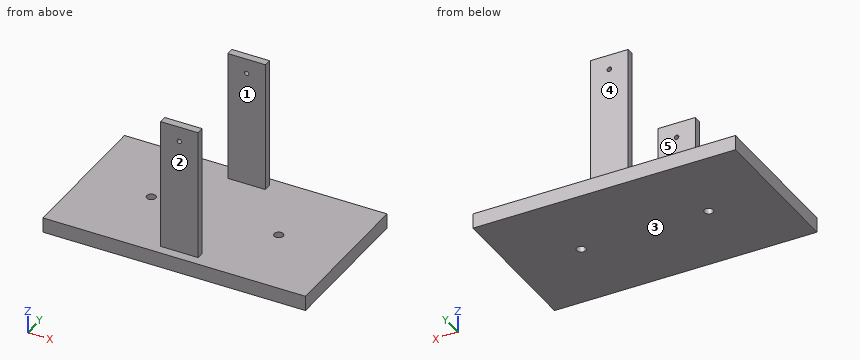
```python
from build123d import *

# Parameters (mm, degrees)
SKETCH_W        = 70
SKETCH_H        = 40
PAD_DEPTH       = 4
SKETCH001_W     = 10
SKETCH001_H     = 2
PAD001_DEPTH    = 35
SKETCH002_R     = 0.6
POCKET_DEPTH    = 37
SKETCH003_R     = 1.2
POCKET001_DEPTH = 5


with BuildPart() as part:
    # Sketch → Pad (new body)
    with BuildSketch(Plane.XY):
        with Locations((35, 20)):
            Rectangle(SKETCH_W, SKETCH_H)
    extrude(amount=PAD_DEPTH)

    # Sketch001 (on Face6 of Pad) → Pad001 (join)
    with BuildSketch(Plane.XY.offset(4)):
        with Locations((35, 36.5)):
            Rectangle(SKETCH001_W, SKETCH001_H)
        with Locations((35, 3.5)):
            Rectangle(SKETCH001_W, SKETCH001_H)
    extrude(amount=PAD001_DEPTH)

    # Sketch002 (on Face8 of Pad001) → Pocket (cut)
    with BuildSketch(Plane.XZ.offset(-2.5)):
        with Locations((35, 35)):
            Circle(SKETCH002_R)
    extrude(amount=-POCKET_DEPTH, mode=Mode.SUBTRACT)

    # Sketch003 (on Face4 of Pocket) → Pocket001 (cut)
    with BuildSketch(Plane(origin=(0, 0, 0), x_dir=(1, 0, 0), z_dir=(0, 0, -1))):
        with Locations((18, -20)):
            Circle(SKETCH003_R)
        with Locations((52, -20)):
            Circle(SKETCH003_R)
    extrude(amount=-POCKET001_DEPTH, mode=Mode.SUBTRACT)


solid = part.part
```
Geometry: final body of the model. Coordinates: model frame, mm. Face numbers are marked on the shaded views. A direction names the side the tool comes from. Coordinates: 2 decimals unless noted, no trailing zeros. Loops run counter-clockwise (first coordinate to the right, second up) from the corner with the lowest first, then second, coordinate; pieces in that order, holes last. Notation, with made-up numbers: M 47.5,-19 L 92.5,-19 A22 cw 92.5,13 Z; hole C -23.75,-14.75 d9. An arc over 180 degrees is marked long. Put each result on its own line as item: value.
(1) Access query for the marked faces 4 and 5. Directions: +Z, -Z, +X, -X, +Y, -Y. A direction counts if a zero-diameter tool reaches every point of the face in a straight line with its end or side. Return the directions, or none.
Answer sheet:
face 4: +Z, +X, -X, +Y
face 5: +Z, +X, -X
(2) Cut plane C-C on x = 33.5. Return the cut outline in (y, z).
Answer sheet:
outline: M 0,0 L 40,0 L 40,4 L 37.5,4 L 37.5,39 L 35.5,39 L 35.5,4 L 4.5,4 L 4.5,39 L 2.5,39 L 2.5,4 L 0,4 Z
(3) First-contact query: pin 1 (5 mm diameter, centred on x = 36.5, z = 27.5, fed in from +Y); pin 2 (10 mm diameter, centred on y = 26, z = 16, fed in from -X); pin 3 (5 mm diameter, centred on x = 35, z = 25, fed in from -Y); pin 4 (0.6 mm diameter, centred on y = 36.5, z = 30, fed in from +X). Flat tips, straight axial feed; report the tip coordinate or a pass-through.
Answer sheet:
pin 1: stops at y = 37.5
pin 2: passes through
pin 3: stops at y = 2.5
pin 4: stops at x = 40
(4) Cut plane A-A on z = 5. Return the cut outline in (x, y), then the cut area to 3 significant figures.
Answer sheet:
outline: M 30,2.5 L 40,2.5 L 40,4.5 L 30,4.5 Z; M 30,35.5 L 40,35.5 L 40,37.5 L 30,37.5 Z
area: 40.0 mm^2
(5) Material intervals for probe 1 along X at (y, z) = (20, 2.7); probe 2 along Y at (x, z) = (36, 33); probe 3 along Y at (x, z) = (52, 3), sorted ascending.
Answer sheet:
probe 1: x = 0 to 16.8, 19.2 to 50.8, 53.2 to 70
probe 2: y = 2.5 to 4.5, 35.5 to 37.5
probe 3: y = 0 to 18.8, 21.2 to 40
(6) Draft query along Y for the marked faces 1, 2 and 3. Return one class per face: pulls with the +Y half, pulls with the -Y half, needs draft (parallel to the pull), parting line crosses it, or undercut.
Answer sheet:
face 1: undercut
face 2: pulls with the -Y half
face 3: needs draft
(7) Cut plane B-B on x = 18. Return the cut outline in (y, z).
Answer sheet:
outline: M 0,0 L 18.8,0 L 18.8,4 L 0,4 Z; M 21.2,0 L 40,0 L 40,4 L 21.2,4 Z
(8) Cut plane D-D on y = 10. Return the cut outline in (x, z).
Answer sheet:
outline: M 0,0 L 70,0 L 70,4 L 0,4 Z
